Model file for the job. Use its own axes, mm. A direction names the side the tool comes from. Coordinates: 2 decimals unless noted, no trailing zeros. Order: outer loops, then holes, each group sorted by start corner. A loop starts at its lowest first (then second) coordinate and runs counter-clockwise, first axis right, second up. Notation, with made-up numbers: (21, -33) -> (31, -33) arc R21 ccw to (31, -15) -> close; hole circle Ø8 at (85, 8). An arc over 180 degrees is marked (long way). Write item = value, one per line. Start each with the question number.
Q1. Cut at A-A, the plane z = 116. List the corners of the cut face in (x, y).
Q2. Mould opens along Y. For faces 4 (the face through (37.04, 30.9, 113.14)), 5 (the face through (0, 6, 99)), 6 (the face through (-29, 3, 13)) say: +Y half, -Y half, draft (parallel to the pull), parting line (faces both ways), or undercut.
Q3. Cut at C-C, the plane y = 17.5. List the corners of the cut face in (x, z).
Q4. Wall check: line 1 (Z direction, x = 27.5, y = 1.6); line 2 (Y direction, x = 38.45, z = 164); line 3 (X direction, y = 9, z = 184.5). Give the ranges that are in metal, low to high. Write a range as from..to.
Q5. Flat gauge pin, fed straight in: pin 1 (20.5 mm diameter, centred on x = 8.5, z = 61.5, fed in from +Y). Where does the tip first touch, or does it go through?
Q6. Cut at B-B, the plane x = -27.5. List the corners of the cut face in (y, z).
Q7. 3-axis set-ups, long thin cutter, end or side, ignore diameter. For faces 1 (the face through (34, 31, 99)), 2 (the face through (-1, 0, 99)), 3 (the face through (37.04, 32.4, 132.37)): which of +Z, -Z, +X, -X, +Y, -Y reach the whole face in a straight line?
Q8. Cut at D-D, the plane z = 185. List the corners of the cut face in (x, y).
from build123d import *

# Parameters (mm, degrees)
EXTRUDE_1_DEPTH     = 200
CUT_EXTRUDE_1_REACH = 82
SKETCH_3_R          = 8
SKETCH_3_R_2        = 3
CUT_EXTRUDE_2_REACH = 58
SKETCH_4_R          = 2.5


with BuildPart() as part:
    # 草图1 → 凸台-拉伸1 (new body)
    with BuildSketch(Plane.XY):
        Polygon((-40, 0), (40, 0), (40, 56), (34, 56), (34, 6), (-34, 6), (-34, 56), (-40, 56), align=None)
    extrude(amount=EXTRUDE_1_DEPTH)

    # 草图3 → 切除-拉伸1 (cut, up to next)
    with BuildSketch(Plane(origin=(40, 0, 0), x_dir=(0, 0, -1), z_dir=(1, 0, 0)), mode=Mode.PRIVATE) as cut_extrude_1_sk1:
        with Locations((-140, 30)):
            Circle(SKETCH_3_R)
    cut_extrude_1_tool1 = extrude(cut_extrude_1_sk1.sketch, amount=-CUT_EXTRUDE_1_REACH, mode=Mode.PRIVATE) & part.part
    add(cut_extrude_1_tool1.solids().sort_by_distance((40, 30, 140))[0], mode=Mode.SUBTRACT)
    # 草图3 → 切除-拉伸1 (cut, up to next)
    with BuildSketch(Plane(origin=(40, 0, 0), x_dir=(0, 0, -1), z_dir=(1, 0, 0)), mode=Mode.PRIVATE) as cut_extrude_1_sk2:
        with Locations((-164, 30)):
            Circle(SKETCH_3_R_2)
    cut_extrude_1_tool2 = extrude(cut_extrude_1_sk2.sketch, amount=-CUT_EXTRUDE_1_REACH, mode=Mode.PRIVATE) & part.part
    add(cut_extrude_1_tool2.solids().sort_by_distance((40, 30, 164))[0], mode=Mode.SUBTRACT)
    # 草图3 → 切除-拉伸1 (cut, up to next)
    with BuildSketch(Plane(origin=(40, 0, 0), x_dir=(0, 0, -1), z_dir=(1, 0, 0)), mode=Mode.PRIVATE) as cut_extrude_1_sk3:
        with Locations((-116, 30)):
            Circle(SKETCH_3_R_2)
    cut_extrude_1_tool3 = extrude(cut_extrude_1_sk3.sketch, amount=-CUT_EXTRUDE_1_REACH, mode=Mode.PRIVATE) & part.part
    add(cut_extrude_1_tool3.solids().sort_by_distance((40, 30, 116))[0], mode=Mode.SUBTRACT)

    # 草图4 → 切除-拉伸2 (cut, up to next)
    with BuildSketch(Plane.XZ, mode=Mode.PRIVATE) as cut_extrude_2_sk1:
        with Locations((-27.5, 185)):
            Circle(SKETCH_4_R)
    cut_extrude_2_tool1 = extrude(cut_extrude_2_sk1.sketch, amount=-CUT_EXTRUDE_2_REACH, mode=Mode.PRIVATE) & part.part
    add(cut_extrude_2_tool1.solids().sort_by_distance((-27.5, 0, 185))[0], mode=Mode.SUBTRACT)
    # 草图4 → 切除-拉伸2 (cut, up to next)
    with BuildSketch(Plane.XZ, mode=Mode.PRIVATE) as cut_extrude_2_sk2:
        with Locations((27.5, 185)):
            Circle(SKETCH_4_R)
    cut_extrude_2_tool2 = extrude(cut_extrude_2_sk2.sketch, amount=-CUT_EXTRUDE_2_REACH, mode=Mode.PRIVATE) & part.part
    add(cut_extrude_2_tool2.solids().sort_by_distance((27.5, 0, 185))[0], mode=Mode.SUBTRACT)
    # 草图4 → 切除-拉伸2 (cut, up to next)
    with BuildSketch(Plane.XZ, mode=Mode.PRIVATE) as cut_extrude_2_sk3:
        with Locations((-27.5, 165)):
            Circle(SKETCH_4_R)
    cut_extrude_2_tool3 = extrude(cut_extrude_2_sk3.sketch, amount=-CUT_EXTRUDE_2_REACH, mode=Mode.PRIVATE) & part.part
    add(cut_extrude_2_tool3.solids().sort_by_distance((-27.5, 0, 165))[0], mode=Mode.SUBTRACT)
    # 草图4 → 切除-拉伸2 (cut, up to next)
    with BuildSketch(Plane.XZ, mode=Mode.PRIVATE) as cut_extrude_2_sk4:
        with Locations((27.5, 165)):
            Circle(SKETCH_4_R)
    cut_extrude_2_tool4 = extrude(cut_extrude_2_sk4.sketch, amount=-CUT_EXTRUDE_2_REACH, mode=Mode.PRIVATE) & part.part
    add(cut_extrude_2_tool4.solids().sort_by_distance((27.5, 0, 165))[0], mode=Mode.SUBTRACT)
    # 草图4 → 切除-拉伸2 (cut, up to next)
    with BuildSketch(Plane.XZ, mode=Mode.PRIVATE) as cut_extrude_2_sk5:
        with Locations((27.5, 35)):
            Circle(SKETCH_4_R)
    cut_extrude_2_tool5 = extrude(cut_extrude_2_sk5.sketch, amount=-CUT_EXTRUDE_2_REACH, mode=Mode.PRIVATE) & part.part
    add(cut_extrude_2_tool5.solids().sort_by_distance((27.5, 0, 35))[0], mode=Mode.SUBTRACT)
    # 草图4 → 切除-拉伸2 (cut, up to next)
    with BuildSketch(Plane.XZ, mode=Mode.PRIVATE) as cut_extrude_2_sk6:
        with Locations((-27.5, 35)):
            Circle(SKETCH_4_R)
    cut_extrude_2_tool6 = extrude(cut_extrude_2_sk6.sketch, amount=-CUT_EXTRUDE_2_REACH, mode=Mode.PRIVATE) & part.part
    add(cut_extrude_2_tool6.solids().sort_by_distance((-27.5, 0, 35))[0], mode=Mode.SUBTRACT)
    # 草图4 → 切除-拉伸2 (cut, up to next)
    with BuildSketch(Plane.XZ, mode=Mode.PRIVATE) as cut_extrude_2_sk7:
        with Locations((27.5, 15)):
            Circle(SKETCH_4_R)
    cut_extrude_2_tool7 = extrude(cut_extrude_2_sk7.sketch, amount=-CUT_EXTRUDE_2_REACH, mode=Mode.PRIVATE) & part.part
    add(cut_extrude_2_tool7.solids().sort_by_distance((27.5, 0, 15))[0], mode=Mode.SUBTRACT)
    # 草图4 → 切除-拉伸2 (cut, up to next)
    with BuildSketch(Plane.XZ, mode=Mode.PRIVATE) as cut_extrude_2_sk8:
        with Locations((-27.5, 15)):
            Circle(SKETCH_4_R)
    cut_extrude_2_tool8 = extrude(cut_extrude_2_sk8.sketch, amount=-CUT_EXTRUDE_2_REACH, mode=Mode.PRIVATE) & part.part
    add(cut_extrude_2_tool8.solids().sort_by_distance((-27.5, 0, 15))[0], mode=Mode.SUBTRACT)


solid = part.part
Here are the results:
q1.outline = (-40, 0) -> (40, 0) -> (40, 27) -> (34, 27) -> (34, 6) -> (-34, 6) -> (-34, 56) -> (-40, 56) -> close; (34, 33) -> (40, 33) -> (40, 56) -> (34, 56) -> close
q2.face_4 = undercut
q2.face_5 = +Y half
q2.face_6 = draft
q3.outline = (-40, 0) -> (-34, 0) -> (-34, 200) -> (-40, 200) -> close; (34, 0) -> (40, 0) -> (40, 200) -> (34, 200) -> close
q4.line_1 = 0..12.5, 17.5..32.5, 37.5..162.5, 167.5..182.5, 187.5..200
q4.line_2 = 0..27, 33..56
q4.line_3 = -40..-34, 34..40
q5.pin_1 = 6
q6.outline = (0, 0) -> (6, 0) -> (6, 12.5) -> (0, 12.5) -> close; (0, 17.5) -> (6, 17.5) -> (6, 32.5) -> (0, 32.5) -> close; (0, 37.5) -> (6, 37.5) -> (6, 162.5) -> (0, 162.5) -> close; (0, 167.5) -> (6, 167.5) -> (6, 182.5) -> (0, 182.5) -> close; (0, 187.5) -> (6, 187.5) -> (6, 200) -> (0, 200) -> close
q7.face_1 = +Z, -Z, +Y
q7.face_2 = +Z, -Z, +X, -X, -Y
q7.face_3 = +X
q8.outline = (-40, 0) -> (-30, 0) -> (-30, 6) -> (-34, 6) -> (-34, 56) -> (-40, 56) -> close; (-25, 0) -> (25, 0) -> (25, 6) -> (-25, 6) -> close; (30, 0) -> (40, 0) -> (40, 56) -> (34, 56) -> (34, 6) -> (30, 6) -> close
